```python
from build123d import *

# Parameters (mm, degrees)
F0_W     = 176
F0_H     = 57.188374
F0_R     = 26
F1_DEPTH = 5
F2_R     = 15
F3_SIZE  = 1


with BuildPart() as f1:
    # F0 (on Front) → F1 (new body)
    with BuildSketch(Plane.XZ):
        with Locations((0, 0.446782)):
            Rectangle(F0_W, F0_H)
        with Locations((-57, 0)):
            Circle(F0_R, mode=Mode.SUBTRACT)
        Circle(F0_R, mode=Mode.SUBTRACT)
        with Locations((57, 0)):
            Circle(F0_R, mode=Mode.SUBTRACT)
        with BuildLine():
            ThreePointArc((99.751152, -28.147405), (98.000731, 1.294425), (88, 29.040969))
            Line((88, 29.040969), (88, -28.147405))
            Line((88, -28.147405), (99.751152, -28.147405))
        make_face()
    extrude(amount=F1_DEPTH)

    # F2
    f2_edges = [f1.edges().sort_by_distance(p)[0] for p in [
        (88, -2.5, 29.040969),
    ]]
    fillet(f2_edges, radius=F2_R)

    # F3
    f3_edges = [f1.edges().sort_by_distance(p)[0] for p in [
        (-83, -5, 0),
        (-26, -5, 0),
        (31, -5, 0),
    ]]
    chamfer(f3_edges, length=F3_SIZE)


solid = f1.part
```
The model under review builds one solid part; all positions refer to its coordinate system, in mm. Coordinates: 2 decimals unless noted, no trailing zeros. Write each loop counter-clockwise with the first axis right and the second up, starting at its lowest first coordinate (ties: lowest second). Pieces come first, ordered by that corner, then holes. Notation, with made-up numbers: (8, 86.25) - (13, 86.25) arc R17 ccw to (13, 106.25) - close; hole circle Ø5 at (38.25, -19). An arc over 180 degrees is marked (long way). Write item = value, one per line.
(1) Consider section A-A, the plane x = -57. Give the boundary of the cut face in (y, z), then the cut area to 3 significant figures.
Result sheet:
outline = (-5, -28.15) - (0, -28.15) - (0, -26) - (-4, -26) - (-5, -27) - close; (-5, 27) - (-4, 26) - (0, 26) - (0, 29.04) - (-5, 29.04) - close
area = 24.9 mm^2
(2) For P1, Ø5, axis at x = -49.5, z = 21, coming from the -Y side, flat-tipped, find the tip position at first contact; note if it passes through.
Result sheet:
P1 = through
(3) Consider section B-B, the plane y = -2.25. Give the boundary of the cut face in (x, z).
Result sheet:
outline = (-88, -28.15) - (99.75, -28.15) arc R103.28 ccw to (92.37, 19.74) arc R15 ccw to (78.5, 29.04) - (-88, 29.04) - close; hole circle Ø52 at (-57, 0); hole circle Ø52 at (0, 0); hole circle Ø52 at (57, 0)
(4) Consider section C-C, the plane z = 24. State how many separate pieces and enclosed holes the cut face has, then the cut area to 3 significant figures.
Result sheet:
separate_pieces = 4
enclosed_holes = 0
area = 581 mm^2
(5) Mouldability with a two-part tool opening along X and no side actions: class faces 1 (the face through (-6, -2, 29.041)), 2 (the face through (31.025, -1.972, 1.143)), 3 (the face through (87, -2.5, 26.4)) as pulls with the +X half, pulls with the -X half, needs draft (parallel to the pull), parting line crosses it, or undercut.
Result sheet:
face_1 = needs draft
face_2 = undercut
face_3 = pulls with the +X half
(6) For line 1 (Z direction, x = 0, y = -1.55); line 2 (X direction, y = -0.75, z = -9.5); line 3 (X direction, y = -2.05, z = -10), list the stretches that pass through material, from the lowest coordinate up. Write a range as [from, to].
Result sheet:
line_1 = [-28.15, -26], [26, 29.04]
line_2 = [-88, -81.2], [-32.8, -24.2], [24.2, 32.8], [81.2, 99.63]
line_3 = [-88, -81], [-33, -24], [24, 33], [81, 99.68]
